Geometry: final body of the model. Coordinates: model frame, mm. A direction names the side the tool comes from. Give positions to 0.01 mm unless a question says otherwise; leave off trailing zeros. Loops run counter-clockwise (first coordinate to the right, second up) from the corner with the lowest first, then second, coordinate; pieces in that order, holes last. Notation, with made-up numbers: M -7,78 L 27,78 A14 ccw 27,105 Z; hole C 85.5,30.5 d10. An arc over 180 degrees is marked long. Put each result on its own line as item: value.
Autodesk Inventor part; units mm, degrees
ref_plane "YZ Plane" through (0, 0, 0) normal (1, 0, 0) x (0, 1, 0)
ref_plane "XZ Plane" through (0, 0, 0) normal (0, 1, 0) x (-1, 0, 0)
sketch "Sketch7" plane through (0, 0, 0) normal (0, 1, 0) x (-1, 0, 0)
  line L0 (0, 0) -> (0, 61.9844)
  line L1 (0, 0) -> (-59.2469, 0) construction
  line L2 (0, 61.9844) -> (-59.2469, 0) construction
  line L3 (0, 61.9844) -> (-64.8494, 0) construction
  line L4 (0, 61.9844) -> (-58.9939, -5.5968) construction
  line L5 (0, 0) -> (0, -61.9844)
  line L6 (0, -61.9844) -> (-59.2469, 0) construction
  line L7 (0, -61.9844) -> (-64.8494, 0) construction
  line L8 (0, -61.9844) -> (-58.9939, 5.5968) construction
  line L9 (-58.9939, 5.5968) -> (-64.8494, 0) construction
  line L10 (-54.1083, 0) -> (-62.8579, -8.363) construction
  line L11 (-54.1083, 0) -> (-38.773, -14.6578) construction
  line L12 (0, -94.3812) -> (0, 132.3969)
  line L13 (-75, -5.9919) -> (-75, 6.008)
  line L14 (105, 0) -> (-105, 0)
  line L15 (-62.0481, 2.6775) -> (-56.4456, -2.6775) construction
  line L16 (-56.4456, 2.6775) -> (-62.0481, -2.6775) construction
  line L17 (-26.151, -15.9303) -> (-40.3783, -15.9303) construction
  line L18 (-40.3783, -15.9303) -> (-40.3783, -12.7539) construction
  line L19 (-40.3783, -12.7539) -> (-26.151, -12.7539) construction
  line L20 (-26.151, -12.7539) -> (-26.151, -15.9303) construction
  point P0 (-75, 0)
  dimension "Roller_Side_difference" = -0.0002
  dimension "d90" = 61.9844
  dimension "d201" = 75
  dimension "d343" = 92.587
  dimension "d344" = 92.588
  dimension "d367" = 8.1
sketch "Sketch1" plane through (0, 0, 0) normal (0, 0, 1) x (1, 0, 0)
  circle A0 centre (0, 0) radius 59.2469 construction
  line L0 (0, 0) -> (59.2469, 0)
  line L1 (0, 0) -> (59.2469, 4.025)
  line L2 (59.2469, 0) -> (59.2469, 4.025)
  circle A1 centre (0, 0) radius 75
  point P0 (56.8, 0)
  dimension "d56" = 59.2469
  dimension "d57" = 4.025
  dimension "d400" = 75
  dimension "d495" = 2.5
  dimension "d496" = 8
  dimension "d531" = 5.5
  dimension "d532" = 5.5
  dimension "d533" = 5.5
  dimension "d537" = 24.5
  dimension "d538" = 3
  dimension "d543" = 5.5
  dimension "d549" = 3
  dimension "d550" = 3
  dimension "d567" = 5.5
  dimension "d568" = 5.5
sketch "Roller1" plane through (0, 0, 0) normal (0, 1, 0) x (-1, 0, 0)
  line L0 (0, 61.9844) -> (-58.9939, -5.5968) construction
  line L1 (0, 61.9844) -> (-64.8494, 0) construction
  line L2 (-54.1083, 0) -> (-38.773, -14.6578) construction
  line L3 (0, -61.9844) -> (-64.8494, 0) construction
  line L4 (-54.0606, 0.0927) -> (-58.9462, -5.5041)
  line L5 (-58.9462, -5.5041) -> (-64.7589, 0.0519)
  line L6 (-64.7589, 0.0519) -> (-59.3884, 5.1851)
  line L7 (-59.3884, 5.1851) -> (-54.0606, 0.0927)
  line L8 (-56.0019, 1.9482) -> (-61.1299, -3.4168)
  line L9 (-61.8526, -2.7261) -> (-56.7246, 2.639)
  point P0 (0, 0)
  dimension "d345" = 0.025
  dimension "d346" = 0.025
  dimension "d347" = 0.1
  dimension "d348" = 0.1
  dimension "d349" = 272.588
  dimension "d350" = 272.587
  dimension "d617" = 0.9997
sketch "Roller2" plane through (0, 0, 0) normal (0, 1, 0) x (-1, 0, 0)
  line L0 (0, -61.9844) -> (-58.9939, 5.5968) construction
  line L1 (-54.1083, 0) -> (-62.8579, -8.363) construction
  line L2 (0, -61.9844) -> (-64.8494, 0) construction
  line L3 (0, 61.9844) -> (-64.8494, 0) construction
  line L4 (-58.9462, 5.5041) -> (-54.1923, 0.0581)
  line L5 (-54.1923, 0.0581) -> (-59.5331, -5.0468)
  line L6 (-59.5331, -5.0468) -> (-64.7589, -0.0519)
  line L7 (-64.7589, -0.0519) -> (-58.9462, 5.5041)
  line L8 (-61.8526, 2.7261) -> (-56.8627, -2.4944)
  line L9 (-61.1297, 3.417) -> (-56.1399, -1.8034)
  point P0 (0, 0)
  dimension "d351" = 0.025
  dimension "d352" = 0.025
  dimension "d354" = 0.1
  dimension "d355" = 92.587
  dimension "d356" = 92.588
  dimension "d370" = 0.1
  dimension "d371" = 1
sketch "Sketch22" plane through (0, 0, 0) normal (0, 1, 0) x (-1, 0, 0)
  line L0 (-31.756, 8.0215) -> (-17.5287, 8.0215) construction
  line L1 (-17.5287, 8.0215) -> (-17.5287, 4.8451) construction
  line L2 (-17.5287, 4.8451) -> (-31.756, 4.8451) construction
  line L3 (-31.756, 4.8451) -> (-31.756, 8.0215) construction
  point P0 (0, 0)
  dimension "Roller_Side_difference" = -0.0002
sketch "Sketch2" plane through (0, 0, 0) normal (0, 1, 0) x (-1, 0, 0)
  line L0 (0, 0) -> (0, 59.2469) construction
  line L1 (0, 0) -> (-59.2469, 0)
  line L2 (0, 0) -> (0, -59.2469)
  line L3 (0, -59.2469) -> (-59.2469, 0) construction
  line L4 (0, 59.2469) -> (-59.2469, 0) construction
  line L5 (-50.488, 53.5552) -> (0, 59.2469) construction
  line L6 (-29.7354, 7.189) -> (0, 59.2469) construction
  line L7 (-29.7354, 7.189) -> (0, -59.2469) construction
  line L8 (-48.8381, -26.254) -> (0, -59.2469) construction
  point P0 (-40.4258, 18.8211)
sketch "Sketch23" plane through (0, 0, 0) normal (0, 1, 0) x (-1, 0, 0)
  line L0 (0, -61.9844) -> (-58.9939, 5.5968) construction
  line L1 (0, -61.9844) -> (-64.8494, 0) construction
  line L2 (0, 61.9844) -> (-58.9939, -5.5968) construction
  line L3 (-58.9939, 5.5968) -> (-64.8494, 0) construction
  line L4 (0, 61.9844) -> (-64.8494, 0) construction
  line L5 (-58.9939, 5.5968) -> (-58.9939, -5.5968) construction
  line L6 (105, 0) -> (-105, 0)
  line L7 (-57.5518, 4.0968) -> (-54.033, 0.0658)
  line L8 (-54.033, -0.0658) -> (-57.5518, -4.0968)
  line L9 (-60.708, 4.0968) -> (-64.9185, 0.0723)
  line L10 (-64.9185, -0.0723) -> (-60.708, -4.0968)
  arc A0 (-64.9185, 0.0723) -> (-64.9185, -0.0723) centre (-64.8494, 0) ccw
  arc A1 (-54.033, -0.0658) -> (-54.033, 0.0658) centre (-54.1083, 0) ccw
  line L11 (-57.5518, 4.0968) -> (-57.5518, 5.5968)
  line L12 (-57.5518, 5.5968) -> (-50, 5.5968)
  line L13 (-50, 5.5968) -> (-50, -5.5968)
  line L14 (-50, -5.5968) -> (-57.5518, -5.5968)
  line L15 (-57.5518, -5.5968) -> (-57.5518, -4.0968)
  line L16 (-60.708, 4.0968) -> (-60.708, 5.5968)
  line L17 (-60.708, 5.5968) -> (-75, 5.5968)
  line L18 (-75, 5.5968) -> (-75, -5.5968)
  line L19 (-60.708, -4.0968) -> (-60.708, -5.5968)
  line L20 (-60.708, -5.5968) -> (-75, -5.5968)
  line L21 (-58.9939, 5.5968) -> (-58.9939, 5.5968)
  line L22 (-58.9939, -5.5968) -> (-58.9939, -5.5968)
  line L23 (0, -94.3812) -> (0, 132.3969)
  line L24 (-64.9941, 0) -> (-75, 0)
  point P0 (0, 0)
  point P1 (-53.9756, 0)
  point P2 (-64.9494, 0)
  point P3 (-75, 0)
  dimension "d378" = 90
  dimension "d379" = 0.1
  dimension "d380" = 0.1
  dimension "d381" = 0.1
  dimension "d382" = 0.1
  dimension "d383" = 0.1
  dimension "d384" = 11.1935
  dimension "d385" = 0
  dimension "d386" = 0
  dimension "d391" = 50
  dimension "d392" = 75
  dimension "d393" = 1.5
  dimension "d394" = 1.5
  dimension "d395" = 1.5
  dimension "d396" = 1.5
revolve "RevRoller1" [suppressed]
fillet "Fillet1" [suppressed]
sketch "Sketch40" plane through (0, 0, -5.231) normal (0, 0, -1) x (-1, 0, 0)
  circle A0 centre (53.5, 0) radius 2.75
  circle A1 centre (0, 0) radius 53.5
  point P0 (53.4293, 2.7491)
  point P1 (53.4293, -2.7491)
  dimension "d585" = 8
  dimension "d587" = 1.75
  dimension "d589" = 3
  dimension "d592" = 2
  dimension "d593" = 12
  dimension "d594" = 12
  dimension "d611" = 360
pattern_circular "Circular Pattern13" [suppressed]
feature "Move Body7" [suppressed]
revolve "Revolution13" [suppressed]
fillet "Fillet3" [suppressed]
pattern_circular "Circular Pattern14" [suppressed]
feature "Move Body6" [suppressed]
revolve "Revolution14" [suppressed]
revolve "OuterRim_Top2" [suppressed]
revolve "OuterRim_Bottom2" add sketch "Sketch23" angle 360 about axis through (0, 0, -10) along (0, 0, 1) contours L6 L18 L17 L16 L9 A0
ref_plane "Work Plane7" through (0, 0, 100) normal (0, 0, 1) x (1, 0, 0)
sketch "Sketch47" plane through (0, 0, 100) normal (0, 0, 1) x (1, 0, 0)
  circle A0 centre (0, 0) radius 75 construction
  circle A1 centre (0, 0) radius 60.708 construction
  circle A2 centre (0, 0) radius 57.5518 construction
  circle A3 centre (0, 0) radius 50 construction
  circle A4 centre (0, 0) radius 69
  point P0 (0, 69)
  dimension "d620" = 69
sketch "Sketch48" plane through (0, 0, 5.5968) normal (0, 0, 1) x (1, 0, 0)
  circle A0 centre (0, 69) radius 2.75
  circle A1 centre (0, 69) radius 1.5
  circle A2 centre (0, 0) radius 69 construction
  dimension "d621" = 3
  dimension "d622" = 5.5
extrude "Extrusion39" cut sketch "Sketch48" against normal blind 5.5968 contours A1
extrude "Extrusion40" cut sketch "Sketch48" against normal blind 3 contours A0 | A1
pattern_circular "Circular Pattern28" count 5 over 360 about axis through (0, 0, 4.8468) along (0, 0, 1) of "Extrusion39", "Extrusion40"
sketch "Sketch49" plane through (0, 0, -5.5968) normal (0, 0, -1) x (-1, 0, 0)
  circle A0 centre (0, 0) radius 69 construction
  circle A1 centre (0, 69) radius 1.5
  line L0 (2.75, 67.4123) -> (0, 65.8246)
  line L1 (0, 65.8246) -> (-2.75, 67.4123)
  line L2 (-2.75, 67.4123) -> (-2.75, 70.5877)
  line L3 (-2.75, 70.5877) -> (0, 72.1754)
  line L4 (0, 72.1754) -> (2.75, 70.5877)
  line L5 (2.75, 70.5877) -> (2.75, 67.4123)
  dimension "d630" = 5.5
  dimension "d631" = 3
extrude "Extrusion41" [suppressed]
extrude "Extrusion42" [suppressed]
pattern_circular "Circular Pattern29" [suppressed]
equation "\"Roller_Side_difference\" = -0.000942deg"
equation "\"Cycloid_Top_Plate_Fasner_Inner\" = 61.25"
equation "\"Cycloid_Top_Plate_Fasner_Outer\" = 85.75"
equation "\"Roller_Hole_Radius\" = 1"
equation "\"Distance_To_Bearing\" = 85.74529"
equation "\"d514\" = 0.2"
properties part number "BottomOuterBearing_TBS"
Item 1: Line query: probe 1 along Y at (x, z) = (-2, 3); probe 2 along X at (y, z) = (64, 3.25); probe 3 along Y at (x, z) = (0, 3.65). Output: solid intervals per line, ascending. Write a range as [from, to].
Output values:
probe 1: [-74.97, -61.82], [61.82, 67.11], [70.89, 74.97]
probe 2: [-39.1, 39.1]
probe 3: [-75, -61.18], [61.18, 66.25], [71.75, 75]
Item 2: Section A-A on y = 0. Output: boundary loops of the cut face in (x, z), then the cut area to 3 significant figures.
Output values:
outline: M -75,0 L -64.95,0 A0.1 cw -64.92,0.07 L -60.71,4.1 L -60.71,5.6 L -75,5.6 Z; M 60.71,4.1 L 64.92,0.07 A0.1 cw 64.95,0 L 75,0 L 75,5.6 L 60.71,5.6 Z
area: 142 mm²
Item 3: Mould query, pull axis X, two halves, no side actions, for faces 1 (the flat face through (1.2, 67.8, 2.597)), 2 (the cylindrical face through (-9.764, -74.362, 2.759)), 3 (the flat face through (0, -61, 5.597)). Classes: pulls with the +X half, pulls with the -X half, needs draft (parallel to the pull), parting line crosses it, or undercut.
Output values:
face 1: undercut
face 2: parting line crosses it
face 3: needs draft
Item 4: Pin query (flat end, axial travel): pin 1 Ø1.8 at (x, y) = (65.62, 21.32) entering from -Z; pin 2 Ø5 at (x, y) = (-65.62, 21.32) entering from -Z; pin 3 Ø1.6 at (x, y) = (65, 20.5) entering from +Z. Return the tip coordinate at first contact, or that it passes through.
Output values:
pin 1: through
pin 2: z = 0
pin 3: z = 2.6
Item 5: Set-up query: faces 4 (the cylindrical face through (-43.116, -56.829, 4.118)), 5 (the cylindrical face through (-13.16, -59.264, 4.857)). Return all of +Z, -Z, +X, -X, +Y, -Y with unobstructed straight access to the full face (end or side cutting, diameter ignored); none if empty.
Output values:
face 4: +Z
face 5: +Z, -Z
